from build123d import *

# Parameters (mm, degrees)
BOSS_EXTRUDE1_DEPTH = 3
CUT_EXTRUDE1_DEPTH  = 1.5
SKETCH3_R           = 1.5
CUT_EXTRUDE2_DEPTH  = 1.5


with BuildPart() as part:
    # Sketch1 → Boss-Extrude1 (new body)
    with BuildSketch(Plane(origin=(0, 0, 0), x_dir=(1, 0, 0), z_dir=(0, 1, 0))):
        Polygon((18.257985868, 29.477662881), (-30.015571152, -6.154677663), (-21.053259688, -85.65107364), (-11.116210191, -84.530784707), (-19.431722538, -10.771546932), (24.196709292, 21.432070044), align=None)
    extrude(amount=BOSS_EXTRUDE1_DEPTH)

    # Sketch2 → Cut-Extrude1 (cut)
    with BuildSketch(Plane(origin=(0, 3, 0), x_dir=(1, 0, 0), z_dir=(0, 1, 0))):
        Polygon((18.257985868, 29.477662881), (24.196709292, 21.432070044), (12.128320037, 12.523984908), (6.189596613, 20.569577745), align=None)
    extrude(amount=-CUT_EXTRUDE1_DEPTH, mode=Mode.SUBTRACT)

    # Sketch3 → Cut-Extrude2 (cut)
    with BuildSketch(Plane(origin=(0, 1.5, 0), x_dir=(1, 0, 0), z_dir=(0, 1, 0))):
        with Locations(Location((17.204551161, 22.485504751, 0), (0, 0, 270))):
            Circle(SKETCH3_R)
    extrude(amount=-CUT_EXTRUDE2_DEPTH, mode=Mode.SUBTRACT)


solid = part.part
Geometry: final body of the model. Coordinates: model frame, mm. A direction names the side the tool comes from. Give positions to 0.01 mm unless a question says otherwise; leave off trailing zeros. Order: outer loops, then holes, each group sorted by start corner. A loop starts at its lowest first (then second) coordinate and runs counter-clockwise, first axis right, second up. Notation, with made-up numbers: (54.5, 60.5) -> (86.5, 60.5) arc R22 ccw to (86.5, 84.5) -> close; hole circle Ø4 at (75.25, -24.5). An arc over 180 degrees is marked (long way). Answer as a JSON object with one key per item and string values.
Q1. Draft query along Z for faces 1 (the flat face through (2.077, 1.479, -5.105)), 2 (the flat face through (-16.15, 1.48, 85.1)), 3 (the flat face through (21.27, 0.74, -25.4)). Return one class per face: released by +Z, released by -Z, zero draft, split by the parting line, or undercut.
Entries:
{"face 1": "undercut", "face 2": "released by +Z", "face 3": "released by -Z"}
Q2. Section B-B (y = 2.5). Output: boundary loops of the cut face in (x, z), plus the area to 3 significant figures.
Entries:
{"outline": "(-30.02, 6.15) -> (6.19, -20.57) -> (12.13, -12.52) -> (-19.43, 10.77) -> (-11.12, 84.53) -> (-21.05, 85.65) -> close", "area": "1,190 mm^2"}
Q3. Section D-D (z = -1.5). Output: boundary loops of the cut face in (x, y), plus the area to 3 significant figures.
Entries:
{"outline": "(-19.65, 0) -> (-2.81, 0) -> (-2.81, 3) -> (-19.65, 3) -> close", "area": "50.5 mm^2"}
Q4. First-contact query: pin 1 (1.5 mm diameter, centred on y = 2, z = 66.5, fed in from +X). Flat tip, straight axial feed; report the tip coordinate or a pass-through.
Entries:
{"pin 1": "stops at x = -13.06"}
Q5. Access query for faces 4 (the flat face through (-15.216, 1.479, 48.167)), 5 (the flat face through (-5.54, 1.48, -11.91)), 6 (the flat face through (15, 1.5, -21)). Directions: +Z, -Z, +X, -X, +Y, -Y. A direction counts if a zero-diameter tool reaches every point of the face in a straight line with its end or side. Return the directions, or none.
Entries:
{"face 4": "+X, +Y, -Y", "face 5": "-Z, -X, +Y, -Y", "face 6": "-Z, +X, +Y"}
Q6. Section A-A (x = -12.5). Output: boundary loops of the cut face in (y, z) (3 decimals), plus the area to 3 significant figures.
Entries:
{"outline": "(0, -6.774) -> (3, -6.774) -> (3, 5.655) -> (0, 5.655) -> close; (0, 72.256) -> (3, 72.256) -> (3, 84.687) -> (0, 84.687) -> close", "area": "74.6 mm^2"}
Q7. Section C-C (x = 8). Output: boundary loops of the cut face in (y, z), plus the area to 3 significant figures.
Entries:
{"outline": "(0, -21.91) -> (1.5, -21.91) -> (1.5, -18.12) -> (3, -18.12) -> (3, -9.48) -> (0, -9.48) -> close", "area": "31.6 mm^2"}
Q8. Material intervals for probe 1 along X at (y, z) = (0.85, -22.5); probe 2 along Y at (x, z) = (16, -24); probe 3 along Z at (x, y) = (-21, 0.9), sorted ascending.
Entries:
{"probe 1": "x = 8.8 to 15.7, 18.7 to 23.41", "probe 2": "y = 0 to 1.5", "probe 3": "z = -0.5 to 85.65"}
